Read the model definition and answer for the solid it produces. Units are mm, in the model's axes. Face numbers are marked on the shaded views. A direction names the side the tool comes from. Give positions to 0.01 mm unless a question says otherwise; leave off trailing zeros. Loops run counter-clockwise (first coordinate to the right, second up) from the corner with the lowest first, then second, coordinate; pieces in that order, holes last. Notation, with made-up numbers: (81.5, 61) - (114.5, 61) arc R12 cw to (114.5, 68) - close; hole circle Ø11 at (-1.75, 7.25). An arc over 180 degrees is marked (long way). Use a Markdown table: item, result. Add a question column.
Item 1: Consider probe 1 along Z at (x, y) = (-8, 47); probe 2 along Y at (x, z) = (-4, 0); probe 3 along X at (y, z) = (44.25, -5.5). Determine where each line is inside the solid, lowest interval first. Write a range as [from, to].
Item 2: For a pull along X with two mould halves and no side action, classify the marked faces 3, 4 and 5 as +X half, -X half, draft (parallel to the pull), parting line (faces both ways), or undercut.
Item 3: A cutting plane is placed at B-B (y = 47). Determine the outline of the cut face in (x, z), plus the area to 3 significant figures.
Item 4: A cutting plane is placed at A-A (z = 0). Determine the outline of the cut face in (x, y).
Item 5: Each of these flat-tipped pins is pushed along its axis until it touches: P1, Ø3.5, axis at y = 47, z = 0, coming from the -X side; P2, Ø6, axis at x = -4, z = -5.5, coming from the +Y side; P3, Ø3, axis at x = -10.5, z = 3.5, coming from the -Y side; P4, Ø6, axis at x = -3.5, y = 43.5, coming from the -Z side. Where does it stop, or does it pass through?
Item 6: Which of the six approach directions +Z, -Z, +X, -X, +Y, -Y give full straight-line access (tool end or side, diameter ignored) to the marked faces 1 and 2?
from build123d import *

# Parameters (mm, degrees)
CHAMFER_1_SIZE  = 1
CHAMFER_1_SIZE2 = 2
CHAMFER_2_SIZE  = 2
CHAMFER_2_SIZE2 = 1


with BuildPart() as part:
    # 草图2 → 旋转1 (revolve)
    with BuildSketch(Plane.XY, mode=Mode.PRIVATE) as revolve_1_sk:
        Polygon((-13, 53), (13, 53), (13, 55), (14.5, 55), (14.5, 49), (-14.5, 49), (-14.5, 55), (-13, 55), align=None)
    revolve(revolve_1_sk.sketch.rotate(Axis((-54.733238043, 47, 0), (1, 0, 0)), 90), axis=Axis((-54.733238043, 47, 0), (1, 0, 0)))

    # 倒角1
    chamfer_1_edges = [part.edges().sort_by_distance(p)[0] for p in [
        (-14.5, 47, -8),
    ]]
    chamfer_1_side = [part.faces().sort_by_distance(p)[0] for p in [
        (-13.75, 47, -8),
    ]]
    chamfer(chamfer_1_edges, length=CHAMFER_1_SIZE, length2=CHAMFER_1_SIZE2, reference=chamfer_1_side[0])

    # 倒角2
    chamfer_2_edges = [part.edges().sort_by_distance(p)[0] for p in [
        (14.5, 47, -8),
    ]]
    chamfer_2_side = [part.faces().sort_by_distance(p)[0] for p in [
        (14.5, 47, -7.77372583),
    ]]
    chamfer(chamfer_2_edges, length=CHAMFER_2_SIZE, length2=CHAMFER_2_SIZE2, reference=chamfer_2_side[0])


solid = part.part
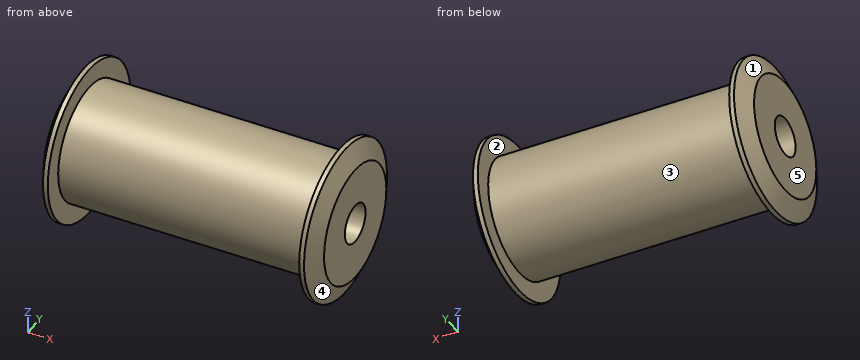
Geometry says:
| question | item | result |
|---|---|---|
| 1 | probe 1 | [-6, -2], [2, 6] |
| 1 | probe 2 | [41, 45], [49, 53] |
| 1 | probe 3 | [-14.43, -13], [13, 14.43] |
| 2 | face 3 | undercut |
| 2 | face 4 | +X half |
| 2 | face 5 | -X half |
| 3 | outline | (-14.5, -6) - (-13.5, -8) - (-13, -8) - (-13, -6) - (13, -6) - (13, -8) - (13.5, -8) - (14.5, -6) - (14.5, -2) - (-14.5, -2) - close; (-14.5, 2) - (14.5, 2) - (14.5, 6) - (13.5, 8) - (13, 8) - (13, 6) - (-13, 6) - (-13, 8) - (-13.5, 8) - (-14.5, 6) - close |
| 3 | area | 240 mm² |
| 4 | outline | (-14.5, 41) - (-13.5, 39) - (-13, 39) - (-13, 41) - (13, 41) - (13, 39) - (13.5, 39) - (14.5, 41) - (14.5, 45) - (-14.5, 45) - close; (-14.5, 49) - (14.5, 49) - (14.5, 53) - (13.5, 55) - (13, 55) - (13, 53) - (-13, 53) - (-13, 55) - (-13.5, 55) - (-14.5, 53) - close |
| 5 | P1 | through |
| 5 | P2 | y = 52.45 |
| 5 | P3 | y = 41.34 |
| 5 | P4 | z = -5.98 |
| 6 | face 1 | -X |
| 6 | face 2 | none |
